Can you work these out from the drawing? Everything is in mm from the part's minimum corner. A direction names the side the tool comes from. Round coordinates to 2 decimals unless told otherwise and drop trailing zeros. Write each loop counter-clockwise with the first axis right and the second up, starting at its lowest first coordinate (ties: lowest second). Pieces come first, ordered by that corner, then holes. Notation, with made-up numbers: (89.25, 31.5) -> (130.25, 31.5) arc R22 cw to (130.25, 53.5) -> close; hole circle Ø11 at (0, 74). An arc over 180 degrees is marked (long way). Put each result on its own line as item: value. Start each with the question number.
1. Suppose I cut it at C-C (y = 20.5). Please give me the cut outline in (x, z), then the cut area to 3 significant figures.
2. We'd pull the mould along Z, two halves only. Please class the marked faces 1, 2, 3 and 4: +Z half, -Z half, draft (parallel to the pull), parting line (faces both ways), or undercut.
3. I need wall thicknesses on probe 1 along Z at (x, y) = (7.4, 23); probe 2 along X at (y, z) = (27.5, 7.25); probe 3 along Y at (x, z) = (21.75, 11.25). Which ranges of each line are inside material? Lowest first, please. Write a range as from..to.
4. Suppose I cut it at D-D (z = 3). Please give me the cut outline in (x, y), then the cut area to 3 significant figures.
5. Suppose I cut it at A-A (y = 8). Please give me the cut outline in (x, z), then the cut area to 3 significant figures.
6. For pin 1 (7.5 mm diameter, centred on x = 9, z = 6.5, fed in from -Y); pin 2 (3.5 mm diameter, centred on y = 16, z = 7.4, fed in from +X); pin 3 (1.5 mm diameter, centred on x = 9, y = 28, fed in from +Z), each with a flat end and sliding along its axis, tell me the tip position at first contact or that it passes through.
7. Which directions (+Z, -Z, +X, -X, +Y, -Y) give clear straight access to the entire face, cutting with the end or side of a thin tool? Please do the marked faces 5 and 6.
8. Suppose I cut it at B-B (x = 20.5). Please give me the cut outline in (y, z).
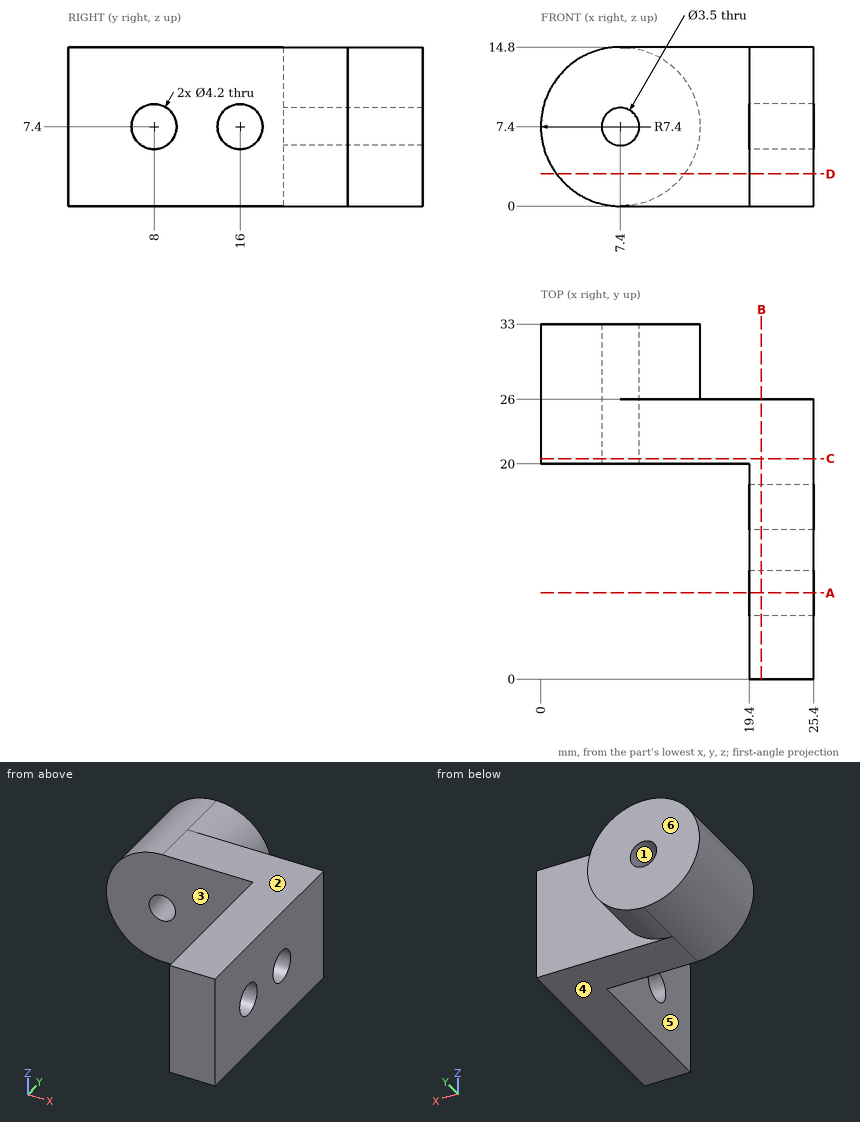
Verdict:
1. outline: (7.4, 0) -> (25.4, 0) -> (25.4, 14.8) -> (7.4, 14.8) arc R7.4 ccw to start; hole circle Ø3.5 at (7.4, 7.4)
1. area: 343 mm^2
2. face 1: undercut
2. face 2: +Z half
2. face 3: draft
2. face 4: -Z half
3. probe 1: z = 0..5.65, 9.15..14.8
3. probe 2: x = 0..5.66, 9.14..14.8
3. probe 3: y = 0..26
4. outline: (1.45, 20) -> (19.4, 20) -> (19.4, 0) -> (25.4, 0) -> (25.4, 26) -> (13.35, 26) -> (13.35, 33) -> (1.45, 33) -> close
4. area: 347 mm^2
5. outline: (19.4, 0) -> (25.4, 0) -> (25.4, 5.3) -> (19.4, 5.3) -> close; (19.4, 9.5) -> (25.4, 9.5) -> (25.4, 14.8) -> (19.4, 14.8) -> close
5. area: 63.6 mm^2
6. pin 1: stops at y = 20
6. pin 2: passes through
6. pin 3: stops at z = 14.75
7. face 5: +Z, -Z, -X, -Y
7. face 6: +Z, -Z, +X, -X, +Y
8. outline: (0, 0) -> (26, 0) -> (26, 14.8) -> (0, 14.8) -> close; hole circle Ø4.2 at (8, 7.4); hole circle Ø4.2 at (16, 7.4)
